Autodesk Inventor part; units mm, degrees
ref_plane "YZ Plane" through (0, 0, 0) normal (1, 0, 0) x (0, 1, 0)
ref_plane "XZ Plane" through (0, 0, 0) normal (0, 1, 0) x (-1, 0, 0)
ref_plane "XY Plane" through (0, 0, 0) normal (0, 0, 1) x (1, 0, 0)
sketch "Sketch1" plane through (0, 0, 0) normal (0, 0, 1) x (1, 0, 0)
  circle A0 centre (0, 0) radius 30
  dimension "d2" = 60
extrude "Extrusion1" add sketch "Sketch1" along normal mid plane 10
sketch "Sketch2" plane through (0, 0, 0) normal (0, 0, 1) x (1, 0, 0)
  line L0 (2.5, 29.8957) -> (-2.5, 29.8957)
  circle A0 centre (0, 0) radius 30
  line L1 (2.5, 30.9866) -> (-2.5, 30.9866)
  line L2 (-2.5, 30.9866) -> (-2.5, 29.8957)
  line L3 (2.5, 29.8957) -> (2.5, 30.9866)
  dimension "d3" = 5
extrude "Extrusion2" cut sketch "Sketch2" along normal mid plane 10 contours L0 A0 picked at (-0.2781, 29.9266)
sketch "Sketch3" plane through (0, 0, 5) normal (0, 0, 1) x (1, 0, 0)
  point P0 (0, 0)
  point P1 (0, 0)
hole "Hole1" at (0, 0, 5) direction (0, 0, -1) diameter 10 end through all
properties part number "pinion" material "Steel, High Strength, Low Alloy"
Geometry check sheet. Reference: the model listing, model coordinates, mm. Round coordinates to 2 decimals unless told otherwise and drop trailing zeros. Order: outer loops, then holes, each group sorted by start corner. A loop starts at its lowest first (then second) coordinate and runs counter-clockwise, first axis right, second up. Notation, with made-up numbers: (51.5, -23.5) -> (87.5, -23.5) arc R32 cw to (87.5, 3.5) -> close; hole circle Ø6 at (76, 24.5). An arc over 180 degrees is marked (long way). Use one line per item in the form item = value.
1. Scan lines: line 1 along Y through (x, z) = (0, 4.25); line 2 along X through (y, z) = (0, 1); line 3 along X through (y, z) = (-3.5, 0). Record each from-to range of solid material in increasing order. Write a range as from..to.
Working result:
line_1 = -30..-5, 5..29.9
line_2 = -30..-5, 5..30
line_3 = -29.8..-3.57, 3.57..29.8
2. Cross-section at A-A, the plane x = 0. Enter the section's corners in (y, z), plus the area to 3 significant figures.
Working result:
outline = (-30, -5) -> (-5, -5) -> (-5, 5) -> (-30, 5) -> close; (5, -5) -> (29.9, -5) -> (29.9, 5) -> (5, 5) -> close
area = 499 mm^2
3. Cross-section at D-D, the plane x = -24. Enter the section's corners in (y, z), plus the area to 3 significant figures.
Working result:
outline = (-18, -5) -> (18, -5) -> (18, 5) -> (-18, 5) -> close
area = 360 mm^2
4. Go/stop test with flat-tipped pins: pin 1 (4 mm diameter, centred on x = -18.5, z = 1, fed in from -Y); pin 2 (2 mm diameter, centred on y = -6, z = 3, fed in from +X); pin 3 (12 mm diameter, centred on x = 2, y = 3, fed in from -Z); pin 4 (2 mm diameter, centred on x = -13.5, z = -3.5, fed in from -Y). Record where each tip stops, or that it passes through.
Working result:
pin_1 = -25.05
pin_2 = 29.58
pin_3 = -5
pin_4 = -27.27
5. Cross-section at B-B, the plane z = 2.5. Enter the section's corners in (x, y).
Working result:
outline = (-2.5, 29.9) arc R30 ccw (long way) to (2.5, 29.9) -> close; hole circle Ø10 at (0, 0)
6. Cross-section at C-C, the plane y = 4. Enter the section's corners in (x, z).
Working result:
outline = (-29.73, -5) -> (-3, -5) -> (-3, 5) -> (-29.73, 5) -> close; (3, -5) -> (29.73, -5) -> (29.73, 5) -> (3, 5) -> close
7. Mould release check, pull along Y, two halves, no side actions. Record for faces 1 (the face through (4.88, 1.08, -0.07)), 2 (the face through (0, 29.896, 0)), 3 (the face through (6, 0, -5)): pulls with the +Y half, pulls with the -Y half, needs draft (parallel to the pull), parting line crosses it, or undercut.
Working result:
face_1 = undercut
face_2 = pulls with the +Y half
face_3 = needs draft
